Work out the finished part from the listing and answer in its coordinate system (mm). A direction names the side the tool comes from. Round coordinates to 2 decimals unless told otherwise and drop trailing zeros. Loops run counter-clockwise (first coordinate to the right, second up) from the corner with the lowest first, then second, coordinate; pieces in that order, holes last. Notation, with made-up numbers: (50.5, 63.25) -> (80.5, 63.25) arc R21 ccw to (80.5, 72.25) -> close; hole circle Ø2 at (28.5, -16). An arc over 180 degrees is marked (long way). Use one line per item in the form item = value.
```python
from build123d import *

# Parameters (mm, degrees)
ESBO_O1_W                = 115.9
ESBO_O1_H                = 75.9
RESSALTO_EXTRUS_O1_DEPTH = 1
ESBO_O2_W                = 125
ESBO_O2_H                = 85
RESSALTO_EXTRUS_O2_DEPTH = 2
ESBO_O3_W                = 71.7
ESBO_O3_H                = 24.6
ESBO_O3_W_2              = 5.1
ESBO_O3_H_2              = 5.1
CORTE_EXTRUS_O1_DEPTH    = 76.640597565


with BuildPart() as part:
    # Esboço1 → Ressalto-extrusão1 (new body)
    with BuildSketch(Plane(origin=(0, 0, 0), x_dir=(1, 0, 0), z_dir=(0, 1, 0))):
        Rectangle(ESBO_O1_W, ESBO_O1_H)
    extrude(amount=RESSALTO_EXTRUS_O1_DEPTH)

    # Esboço2 → Ressalto-extrusão2 (add)
    with BuildSketch(Plane(origin=(0, 1, 0), x_dir=(1, 0, 0), z_dir=(0, 1, 0))):
        Rectangle(ESBO_O2_W, ESBO_O2_H)
    extrude(amount=RESSALTO_EXTRUS_O2_DEPTH)

    # Esboço3 → Corte-extrusão1 (cut, through all)
    with BuildSketch(Plane(origin=(0, 3, 0), x_dir=(1, 0, 0), z_dir=(0, 1, 0))):
        with Locations((0, 15.2)):
            Rectangle(ESBO_O3_W, ESBO_O3_H)
        with Locations((-39.95, -19.95)):
            Rectangle(ESBO_O3_W_2, ESBO_O3_H_2)
    extrude(amount=-CORTE_EXTRUS_O1_DEPTH, mode=Mode.SUBTRACT)


solid = part.part
```
(1) Find section A-A, the plane z = -26. Write down the section's boundary in (x, y).
Completed:
outline = (-62.5, 1) -> (-57.95, 1) -> (-57.95, 0) -> (-35.85, 0) -> (-35.85, 3) -> (-62.5, 3) -> close; (35.85, 0) -> (57.95, 0) -> (57.95, 1) -> (62.5, 1) -> (62.5, 3) -> (35.85, 3) -> close
(2) Consider L1, parallel to Z at x = -4.5, y = 0.85; L2, parallel to Z at x = 14, y = 1.3; L3, parallel to X at y = 1.7, z = 22. Determine where each line is inside the solid, lowest interval first.
Completed:
L1 = -37.95 to -27.5, -2.9 to 37.95
L2 = -42.5 to -27.5, -2.9 to 42.5
L3 = -62.5 to -42.5, -37.4 to 62.5
(3) For faces 3 (the flat face through (-37.4, 2, 20)), 4 (the flat face through (-1, 0, -1)), determine the directions among +Z, -Z, +X, -X, +Y, -Y from which every point of the face is accessible in a straight line to the end or side of a thin tool.
Completed:
face_3 = +Y, -Y
face_4 = +Z, -Z, +X, -X, -Y
(4) Find section B-B, the plane x = 31. Write down the section's boundary in (y, z), then the cut area to 3 significant figures.
Completed:
outline = (0, -37.95) -> (1, -37.95) -> (1, -42.5) -> (3, -42.5) -> (3, -27.5) -> (0, -27.5) -> close; (0, -2.9) -> (3, -2.9) -> (3, 42.5) -> (1, 42.5) -> (1, 37.95) -> (0, 37.95) -> close
area = 172 mm2
(5) Find section D-D, the plane x = 46. Write down the section's boundary in (y, z).
Completed:
outline = (0, -37.95) -> (1, -37.95) -> (1, -42.5) -> (3, -42.5) -> (3, 42.5) -> (1, 42.5) -> (1, 37.95) -> (0, 37.95) -> close
(6) For a pull along Z with two mould halves and no side action, classify faces 1 (the flat face through (-1, 3, -1)), 2 (the flat face through (-42.5, 2, 20)) as +Z half, -Z half, draft (parallel to the pull), parting line (faces both ways), or undercut.
Completed:
face_1 = draft
face_2 = undercut
(7) Find section C-C, the plane y = 2.3. Write down the section's boundary in (x, z).
Completed:
outline = (-62.5, -42.5) -> (62.5, -42.5) -> (62.5, 42.5) -> (-62.5, 42.5) -> close; hole (-42.5, 17.4) -> (-37.4, 17.4) -> (-37.4, 22.5) -> (-42.5, 22.5) -> close; hole (-35.85, -27.5) -> (35.85, -27.5) -> (35.85, -2.9) -> (-35.85, -2.9) -> close
(8) Given P1, Ø1.5, axis at x = 41, y = 0.5, coming from the -Z side, flat-ended and moving along its own axis, determine where the tip first touches the part or whether it passes through.
Completed:
P1 = -42.5
